Design review of the part built by this model. Coordinates are the model's own, in mm. Coordinates: 2 decimals unless noted, no trailing zeros. Loops run counter-clockwise (first coordinate to the right, second up) from the corner with the lowest first, then second, coordinate; pieces in that order, holes last. Notation, with made-up numbers: (60.25, 48) -> (119.25, 48) arc R12 cw to (119.25, 56) -> close; hole circle Ø7 at (5.5, 69). An arc over 180 degrees is marked (long way). Use one line per item in the form item = value. Start each with the question number.
1. The part is to be moulded in two halves that separate along Y. For faces 1 (the face through (-4, 3, 0)), 2 (the face through (-4, -215.9, 10)), 3 (the face through (-4, 3, 12.7)), say which applies: released by +Y, released by -Y, zero draft, split by the parting line, or undercut.
2. Consider section B-B (x = 180.5). State the section outline as (y, z) points, then the cut area to 3 significant figures.
3. Wall thickness on line 1 (X direction, y = -72, z = 12.75); line 2 (Z direction, x = 61, y = 4); line 3 (X direction, y = -4.5, z = 14.75): over which ranges is each line inside the solid? List them lowest first. Write a range as from..to.
4. Consider section A-A (y = 56.5). State the section outline as (x, z) points, then the cut area to 3 significant figures.
5. For pin 1 (8 mm diameter, centred on x = -159.5, y = 112.5, fed in from -Z); pin 2 (12 mm diameter, centred on x = -39, y = 93, fed in from +Z), all flat-tipped, find the tip position at first contact; note any pin that passes through.
from build123d import *

# Parameters (mm, degrees)
F0_W         = 584.2
F0_H         = 431.8
F1_DEPTH     = 12.7
F2_W         = 584.2
F2_H         = 431.8
F2_W_2       = 558.8
F2_H_2       = 406.4
F3_DEPTH     = 7.62
F4_T4_DEPTH  = 558.8
F4_T9_DEPTH  = 406.4
F4_T14_DEPTH = 558.8
F4_T19_DEPTH = 406.4
F4_T25_DEPTH = 439.0603739472
F4_T31_DEPTH = 591.4603739472
F4_T40_DEPTH = 591.4603739472
F4_T46_DEPTH = 439.0603739472
F4_T55_DEPTH = 439.0603739472
F4_T61_DEPTH = 591.4603739472
F4_T70_DEPTH = 439.0603739472
F4_T76_DEPTH = 591.4603739472


# Not quite as in the source:
# - a fillet or chamfer that OpenCascade refuses, or shapes differently, is made with other operations: its cross-section is extruded or revolved along the edge and cut away or added


with BuildPart() as f1:
    # F0 (on Top) → F1 (new body)
    with BuildSketch(Plane.XY):
        Rectangle(F0_W, F0_H)
    extrude(amount=F1_DEPTH)

    # F2 (on face) → F3 (join)
    with BuildSketch(Plane.XY.offset(12.7)):
        Rectangle(F2_W, F2_H)
        Rectangle(F2_W_2, F2_H_2, mode=Mode.SUBTRACT)
    extrude(amount=F3_DEPTH)

    # F4: chamfer of 12.7 on 4 edges, made by hand


with BuildPart() as f4_tool2:
    # F4_s3 → F4_t4 (new body)
    with BuildSketch(Plane.YZ.offset(-279.4)):
        Polygon((215.9, 20.32), (203.2, 7.62), (203.2, 20.32), align=None)
    extrude(amount=F4_T4_DEPTH)

    split(bisect_by=Plane.XY.offset(12.7), keep=Keep.TOP)


with BuildPart() as f1_1:
    add(f1.part)

    # F4_t1: cut F4_tool2
    add(f4_tool2.part, mode=Mode.SUBTRACT)


with BuildPart() as f4_tool7:
    # F4_s8 → F4_t9 (new body)
    with BuildSketch(Plane.XZ.offset(-203.2)):
        Polygon((292.1, 20.32), (279.4, 7.62), (279.4, 20.32), align=None)
    extrude(amount=F4_T9_DEPTH)

    split(bisect_by=Plane.XY.offset(12.7), keep=Keep.TOP)


with BuildPart() as f1_2:
    add(f1_1.part)

    # F4_t6: cut F4_tool7
    add(f4_tool7.part, mode=Mode.SUBTRACT)


with BuildPart() as f4_tool12:
    # F4_s13 → F4_t14 (new body)
    with BuildSketch(Plane.YZ.offset(279.4)):
        Polygon((-215.9, 20.32), (-203.2, 7.62), (-203.2, 20.32), align=None)
    extrude(amount=-F4_T14_DEPTH)

    split(bisect_by=Plane.XY.offset(12.7), keep=Keep.TOP)


with BuildPart() as f1_3:
    add(f1_2.part)

    # F4_t11: cut F4_tool12
    add(f4_tool12.part, mode=Mode.SUBTRACT)


with BuildPart() as f4_tool17:
    # F4_s18 → F4_t19 (new body)
    with BuildSketch(Plane.XZ.offset(203.2)):
        Polygon((-292.1, 20.32), (-279.4, 7.62), (-279.4, 20.32), align=None)
    extrude(amount=-F4_T19_DEPTH)

    split(bisect_by=Plane.XY.offset(12.7), keep=Keep.TOP)


with BuildPart() as f1_4:
    add(f1_3.part)

    # F4_t16: cut F4_tool17
    add(f4_tool17.part, mode=Mode.SUBTRACT)


with BuildPart() as f4_tool23:
    # F4_s24 → F4_t25 (new body)
    with BuildSketch(Plane.XZ.offset(203.2)):
        Polygon((-292.1, 20.32), (-279.4, 7.62), (-279.4, 20.32), align=None)
    extrude(amount=-F4_T25_DEPTH)

    split(bisect_by=Plane.XZ.offset(-215.9), keep=Keep.TOP)

    split(bisect_by=Plane.XY.offset(12.7), keep=Keep.TOP)

    split(bisect_by=Plane.XZ.offset(-203.2), keep=Keep.BOTTOM)


with BuildPart() as f4_tool29:
    # F4_s30 → F4_t31 (new body)
    with BuildSketch(Plane.YZ.offset(-312.0603739472)):
        Polygon((215.9, 20.32), (203.2, 7.62), (203.2, 20.32), align=None)
    extrude(amount=F4_T31_DEPTH)

    split(bisect_by=Plane.XY.offset(12.7), keep=Keep.TOP)

    split(bisect_by=Plane.YZ.offset(-279.4), keep=Keep.BOTTOM)

    split(bisect_by=Plane.YZ.offset(-292.1), keep=Keep.TOP)


with BuildPart() as f4_tool23_1:
    add(f4_tool23.part)

    # F4_t35: intersect F4_tool29
    add(f4_tool29.part, mode=Mode.INTERSECT)


with BuildPart() as f1_5:
    add(f1_4.part)

    # F4_t21: cut F4_tool23
    add(f4_tool23_1.part, mode=Mode.SUBTRACT)


with BuildPart() as f4_tool38:
    # F4_s39 → F4_t40 (new body)
    with BuildSketch(Plane.YZ.offset(-279.4)):
        Polygon((215.9, 20.32), (203.2, 7.62), (203.2, 20.32), align=None)
    extrude(amount=F4_T40_DEPTH)

    split(bisect_by=Plane.YZ.offset(292.1), keep=Keep.BOTTOM)

    split(bisect_by=Plane.XY.offset(12.7), keep=Keep.TOP)

    split(bisect_by=Plane.YZ.offset(279.4), keep=Keep.TOP)


with BuildPart() as f4_tool44:
    # F4_s45 → F4_t46 (new body)
    with BuildSketch(Plane.XZ.offset(-235.8603739472)):
        Polygon((292.1, 20.32), (279.4, 7.62), (279.4, 20.32), align=None)
    extrude(amount=F4_T46_DEPTH)

    split(bisect_by=Plane.XZ.offset(-215.9), keep=Keep.TOP)

    split(bisect_by=Plane.XY.offset(12.7), keep=Keep.TOP)

    split(bisect_by=Plane.XZ.offset(-203.2), keep=Keep.BOTTOM)


with BuildPart() as f4_tool38_1:
    add(f4_tool38.part)

    # F4_t50: intersect F4_tool44
    add(f4_tool44.part, mode=Mode.INTERSECT)


with BuildPart() as f1_6:
    add(f1_5.part)

    # F4_t36: cut F4_tool38
    add(f4_tool38_1.part, mode=Mode.SUBTRACT)


with BuildPart() as f4_tool53:
    # F4_s54 → F4_t55 (new body)
    with BuildSketch(Plane.XZ.offset(-203.2)):
        Polygon((292.1, 20.32), (279.4, 7.62), (279.4, 20.32), align=None)
    extrude(amount=F4_T55_DEPTH)

    split(bisect_by=Plane.XZ.offset(215.9), keep=Keep.BOTTOM)

    split(bisect_by=Plane.XZ.offset(203.2), keep=Keep.TOP)

    split(bisect_by=Plane.XY.offset(12.7), keep=Keep.TOP)


with BuildPart() as f4_tool59:
    # F4_s60 → F4_t61 (new body)
    with BuildSketch(Plane.YZ.offset(312.0603739472)):
        Polygon((-215.9, 20.32), (-203.2, 7.62), (-203.2, 20.32), align=None)
    extrude(amount=-F4_T61_DEPTH)

    split(bisect_by=Plane.YZ.offset(292.1), keep=Keep.BOTTOM)

    split(bisect_by=Plane.XY.offset(12.7), keep=Keep.TOP)

    split(bisect_by=Plane.YZ.offset(279.4), keep=Keep.TOP)


with BuildPart() as f4_tool53_1:
    add(f4_tool53.part)

    # F4_t65: intersect F4_tool59
    add(f4_tool59.part, mode=Mode.INTERSECT)


with BuildPart() as f1_7:
    add(f1_6.part)

    # F4_t51: cut F4_tool53
    add(f4_tool53_1.part, mode=Mode.SUBTRACT)


with BuildPart() as f4_tool68:
    # F4_s69 → F4_t70 (new body)
    with BuildSketch(Plane.XZ.offset(235.8603739472)):
        Polygon((-292.1, 20.32), (-279.4, 7.62), (-279.4, 20.32), align=None)
    extrude(amount=-F4_T70_DEPTH)

    split(bisect_by=Plane.XZ.offset(215.9), keep=Keep.BOTTOM)

    split(bisect_by=Plane.XZ.offset(203.2), keep=Keep.TOP)

    split(bisect_by=Plane.XY.offset(12.7), keep=Keep.TOP)


with BuildPart() as f4_tool74:
    # F4_s75 → F4_t76 (new body)
    with BuildSketch(Plane.YZ.offset(279.4)):
        Polygon((-215.9, 20.32), (-203.2, 7.62), (-203.2, 20.32), align=None)
    extrude(amount=-F4_T76_DEPTH)

    split(bisect_by=Plane.XY.offset(12.7), keep=Keep.TOP)

    split(bisect_by=Plane.YZ.offset(-279.4), keep=Keep.BOTTOM)

    split(bisect_by=Plane.YZ.offset(-292.1), keep=Keep.TOP)


with BuildPart() as f4_tool68_1:
    add(f4_tool68.part)

    # F4_t80: intersect F4_tool74
    add(f4_tool74.part, mode=Mode.INTERSECT)


with BuildPart() as f1_8:
    add(f1_7.part)

    # F4_t66: cut F4_tool68
    add(f4_tool68_1.part, mode=Mode.SUBTRACT)


solid = f1_8.part
Geometry check:
q1.face_1 = zero draft
q1.face_2 = released by -Y
q1.face_3 = undercut
q2.outline = (-215.9, 0) -> (215.9, 0) -> (215.9, 20.32) -> (208.28, 12.7) -> (-208.28, 12.7) -> (-215.9, 20.32) -> close
q2.area = 5,540 mm²
q3.line_1 = -292.1..-284.53, 284.53..292.1
q3.line_2 = 0..12.7
q3.line_3 = -292.1..-286.53, 286.53..292.1
q4.outline = (-292.1, 0) -> (292.1, 0) -> (292.1, 20.32) -> (284.48, 12.7) -> (-284.48, 12.7) -> (-292.1, 20.32) -> close
q4.area = 7,480 mm²
q5.pin_1 = 0
q5.pin_2 = 12.7
